Source: CAD feature listing. Evaluate the final solid. Frame: model axes, mm. A direction names the side the tool comes from. Round coordinates to 2 decimals unless told otherwise and drop trailing zeros. Put each result on its own line as item: value. Start each with the question number.
```python
from build123d import *

# Parameters (mm, degrees)
PAD007_DEPTH       = 10
SKETCH012_R        = 2.5
POCKET003_DEPTH    = 425.270426
POLARPATTERN_COUNT = 3


with BuildPart() as part:
    # Sketch011 → Pad007 (new body)
    with BuildSketch(Plane.XY):
        Polygon((-51.516335, 60.77109), (51.516335, 60.77109), (78.387475, 14.22891), (26.87114, -75), (-26.87114, -75), (-78.387475, 14.22891), align=None)
    extrude(amount=PAD007_DEPTH)

    # Sketch012 → Pocket003 (cut, through all)
    with BuildSketch(Plane.XY):
        with Locations((-35, 50.77109)):
            Circle(SKETCH012_R)
        with Locations((35, 50.77109)):
            Circle(SKETCH012_R)
        with Locations((-35, 30.77109)):
            Circle(SKETCH012_R)
        with Locations((35, 30.77109)):
            Circle(SKETCH012_R)
        Polygon((23.226799, 60.77109), (12.228239, 45.7), (-12.228239, 45.7), (-23.226799, 60.77109), align=None)
    pocket003 = extrude(amount=POCKET003_DEPTH, mode=Mode.SUBTRACT)

    # PolarPattern: Pocket003 ×3 about axis
    polarpattern_axis = Axis((0, 0, 0), (0, 0, 1))
    for i in range(1, POLARPATTERN_COUNT):
        add(pocket003.rotate(polarpattern_axis, i * 360 / POLARPATTERN_COUNT), mode=Mode.SUBTRACT)


solid = part.part
```
(1) Ray query, line 1 along Y through (x, z) = (-35, 6.75); line 2 along X through (y, z) = (32, 5.25); line 3 along X through (y, z) = (-46.5, 5.25). Return the intervals inside material, ascending.
(2) Access query for faces 1 (the cylindrical face through (-25.125, -53.588, 4.93)), 2 (the flat face through (-17.65, 53.13, 4.93)), 3 (the flat face through (-37.187, -41.851, 4.93)), 4 (the flat face through (39.49, -23, 4.93)). Directions: +Z, -Z, +X, -X, +Y, -Y. A direction counts if a zero-diameter tool reaches every point of the face in a straight line with its end or side. Return the directions, or none.
(3) Contact query for flat-ended pins moving along their axis: P1, Ø1.5, axis at x = 48, z = 9, coming from the -Y side; P2, Ø4, axis at x = -44.15, y = 14.93, coming from the -Z side; P3, Ø6, axis at y = -45, z = 1, coming from the -X side; P4, Ø1.5, axis at y = -29, z = 1.5, coming from the +X side. Output: stop coordinate, or through.
(4) Section query A-A (z = 1.5). Count the separate pieces of the cut face and the enclosed holes in it, and give its area (3 significant figures).
(5) Pull-direction query (Y, two-part tool) for faces 5 (the flat face through (-71.216, 1.808, 4.93)), 6 (the flat face through (64.76, 37.83, 4.93)), 7 (the cylindrical face through (-32.69, 29.81, 4.93)); classes: +Y half, -Y half, draft (parallel to the pull), parting line (faces both ways), or undercut.
Entries:
1. line 1: -60.92 to -36.91, -30.78 to 28.27, 33.27 to 48.27, 53.27 to 60.77
1. line 2: -68.13 to -37.18, -32.82 to 32.82, 37.18 to 68.13
1. line 3: -39.24 to -11.52, -6.78 to 6.78, 11.52 to 39.24
2. face 1: +Z, -Z
2. face 2: +Z, -Z, +Y
2. face 3: +Z, -Z, -X
2. face 4: +Z, -Z, +X
3. P1: y = -12.09
3. P2: through
3. P3: x = -39.91
3. P4: x = 36.46
4. separate pieces: 1
4. enclosed holes: 12
4. area: 13,600 mm2
5. face 5: -Y half
5. face 6: +Y half
5. face 7: undercut
